Check sheet for the modelled part. Datum: model origin and axes. Units: mm. A direction names the side the tool comes from. Round coordinates to 2 decimals unless told otherwise and drop trailing zeros. Order: outer loops, then holes, each group sorted by start corner. A loop starts at its lowest first (then second) coordinate and runs counter-clockwise, first axis right, second up.
Q1. Cross-section at B-B on y = -12.5. Record the cut outline in (x, z), then the cut area to 3 significant figures.
Q2. Cross-section at A-A on x = 40. Record the cut outline in (y, z), then the cut area to 3 significant figures.
Q3. Scan lines: probe 1 along Z at (x, y) = (40, -13); probe 2 along Z at (x, y) = (42.5, -35.5); probe 3 along Z at (x, y) = (36.5, -9). Record each from-to range of solid material in increasing order.
Q4. Depth check by flat-ended pin: P1, Ø1.5, axis at x = 24, y = -31.5, coming from the -Z side; P2, Ø8, axis at x = 40, z = -24, coming from the -Y side; P3, Ø10, axis at x = 46.5, z = -14, coming from the -Y side; P4, Ø5, axis at x = 42.5, y = -30.5, coming from the -Z side. Enter the tip coordinate at first touch or a pass-through.
Q5. Mould release check, pull along X, two halves, no side actions. Record for faces 1 (the flat face through (26, -18, 0)), 2 (the cylindrical face through (0.86, -39.1, -15.72)), 3 (the cylindrical face through (36, -11, -27)): +X half, -X half, draft (parallel to the pull), parting line (faces both ways), or undercut.
Q6. Set-up check for faces 4 (the flat face through (54, -30, -11)), 5 (the cylindrical face through (54.1, -39.14, -6.01)): record each of +Z, -Z, +X, -X, +Y, -Y from which the full face is reachable in a straight line by a thin tool's end or side.
Q7. Cross-section at C-C on z = -24. Record the cut outline in (x, y), then the cut area to 3 significant figures.
Q8. Cross-section at D-D on y = -34.5. Record the cut outline in (x, z).
from build123d import *

# Parameters (mm, degrees)
F0_W         = 55
F0_H         = 32
F1_DEPTH     = 40
F2_W         = 30
F2_H         = 18
F3_DEPTH     = 20
F4_R         = 5
F5_DEPTH     = 22.001
F6_SIZE      = 2
F7_T1_DEPTH  = 36
F7_T3_DEPTH  = 45
F7_T5_DEPTH  = 68
F7_T7_DEPTH  = 23
F7_T12_DEPTH = 34.2132034356
F7_T17_DEPTH = 24.2132034356
F7_T22_DEPTH = 13.4214256026
F7_T29_DEPTH = 34.2132034356
F7_T33_DEPTH = 13.4214256026
F7_T40_DEPTH = 13.4214256026
F7_T44_DEPTH = 24.2132034356


# Not quite as in the source:
# - a fillet or chamfer that OpenCascade refuses, or shapes differently, is made with other operations: its cross-section is extruded or revolved along the edge and cut away or added


with BuildPart() as f1:
    # F0 (on Front) → F1 (new body)
    with BuildSketch(Plane.XZ):
        with Locations((27.5, -16)):
            Rectangle(F0_W, F0_H)
    extrude(amount=F1_DEPTH)

    # F2 (on face) → F3 (cut)
    with BuildSketch(Plane(origin=(0, 0, -32), x_dir=(1, 0, 0), z_dir=(0, 0, -1))):
        with Locations((40, 31)):
            Rectangle(F2_W, F2_H)
    extrude(amount=-F3_DEPTH, mode=Mode.SUBTRACT)

    # F4 (on face) → F5 (cut, through all)
    with BuildSketch(Plane.XZ.offset(22)):
        with Locations((40, -24)):
            Circle(F4_R)
    extrude(amount=-F5_DEPTH, mode=Mode.SUBTRACT)

    # F6
    f6_edges = [f1.edges().sort_by_distance(p)[0] for p in [
        (25, -40, -22),
        (25, -31, -32),
        (25, -31, -12),
        (55, -31, -12),
        (40, -40, -12),
        (55, -20, 0),
        (0, -20, -32),
    ]]
    chamfer(f6_edges, length=F6_SIZE)

    # F7: fillet of radius 3 on 7 edges, made by hand

    # F7_s2 → F7_t1 (cut)
    with BuildSketch(Plane.YZ.offset(-5.5)):
        with BuildLine():
            ThreePointArc((-40, -29), (-39.1213203436, -31.1213203436), (-37, -32))
            Line((-37, -32), (-40, -32))
            Line((-40, -32), (-40, -29))
        make_face()
    extrude(amount=F7_T1_DEPTH, mode=Mode.SUBTRACT)

    # F7_s4 → F7_t3 (cut)
    with BuildSketch(Plane.XY.offset(-37.5)):
        with BuildLine():
            ThreePointArc((0, -37), (0.8786796564, -39.1213203436), (3, -40))
            Line((3, -40), (0, -40))
            Line((0, -40), (0, -37))
        make_face()
    extrude(amount=F7_T3_DEPTH, mode=Mode.SUBTRACT)

    # F7_s6 → F7_t5 (cut)
    with BuildSketch(Plane.YZ.offset(-7.5)):
        with BuildLine():
            ThreePointArc((-37, 0), (-39.1213203436, -0.8786796564), (-40, -3))
            Line((-40, -3), (-40, 0))
            Line((-40, 0), (-37, 0))
        make_face()
    extrude(amount=F7_T5_DEPTH, mode=Mode.SUBTRACT)

    # F7_s8 → F7_t7 (cut)
    with BuildSketch(Plane.XY.offset(-17.5)):
        with BuildLine():
            ThreePointArc((52, -40), (54.1213203436, -39.1213203436), (55, -37))
            Line((55, -37), (55, -40))
            Line((55, -40), (52, -40))
        make_face()
    extrude(amount=F7_T7_DEPTH, mode=Mode.SUBTRACT)


with BuildPart() as f7_tool10:
    # F7_s11 → F7_t12 (new body)
    with BuildSketch(Plane.YZ.offset(58.1066017178)):
        with BuildLine():
            ThreePointArc((-40, -8.7573593129), (-39.7716385975, -9.90540961), (-39.1213203436, -10.8786796564))
            Line((-39.1213203436, -10.8786796564), (-40, -10))
            Line((-40, -10), (-40, -8.7573593129))
        make_face()
    extrude(amount=-F7_T12_DEPTH)

    split(bisect_by=Plane(origin=(25.6666666667, -25.6666666667, -25.6666666667), x_dir=(0.7071067812, 0.7071067812, 0), z_dir=(0.5773502692, -0.5773502692, -0.5773502692)), keep=Keep.TOP)


with BuildPart() as f1_1:
    add(f1.part)

    # F7_t9: cut F7_tool10
    add(f7_tool10.part, mode=Mode.SUBTRACT)


with BuildPart() as f7_tool15:
    # F7_s16 → F7_t17 (new body)
    with BuildSketch(Plane.XY.offset(-35.1066017178)):
        with BuildLine():
            ThreePointArc((21.7573593129, -40), (22.90540961, -39.7716385975), (23.8786796564, -39.1213203436))
            Line((23.8786796564, -39.1213203436), (23, -40))
            Line((23, -40), (21.7573593129, -40))
        make_face()
    extrude(amount=F7_T17_DEPTH)

    split(bisect_by=Plane(origin=(25.6666666667, -25.6666666667, -25.6666666667), x_dir=(0.7071067812, 0.7071067812, 0), z_dir=(0.5773502692, -0.5773502692, -0.5773502692)), keep=Keep.TOP)


with BuildPart() as f1_2:
    add(f1_1.part)

    # F7_t14: cut F7_tool15
    add(f7_tool15.part, mode=Mode.SUBTRACT)


with BuildPart() as f7_tool20:
    # F7_s21 → F7_t22 (new body)
    with BuildSketch(Plane(origin=(11.2451905284, 0, 11.2451905284), x_dir=(0, 1, 0), z_dir=(-0.7071067812, 0, -0.7071067812))):
        with BuildLine():
            ThreePointArc((-40, 24.6100366333), (-39.6642215019, 25.9891391634), (-38.7320508076, 27.0595263761))
            Line((-38.7320508076, 27.0595263761), (-40, 26.1629509039))
            Line((-40, 26.1629509039), (-40, 24.6100366333))
        make_face()
    extrude(amount=F7_T22_DEPTH)

    split(bisect_by=Plane(origin=(0, -25, -25), x_dir=(1, 0, 0), z_dir=(0, -0.7071067812, -0.7071067812)), keep=Keep.TOP)

    split(bisect_by=Plane(origin=(31.5, -31.5, 0), x_dir=(0, 0, 1), z_dir=(0.7071067812, -0.7071067812, 0)), keep=Keep.TOP)


with BuildPart() as f1_3:
    add(f1_2.part)

    # F7_t19: cut F7_tool20
    add(f7_tool20.part, mode=Mode.SUBTRACT)


with BuildPart() as f7_tool27:
    # F7_s28 → F7_t29 (new body)
    with BuildSketch(Plane.YZ.offset(58.1066017178)):
        with BuildLine():
            ThreePointArc((-40, -8.7573593129), (-39.7716385975, -9.90540961), (-39.1213203436, -10.8786796564))
            Line((-39.1213203436, -10.8786796564), (-40, -10))
            Line((-40, -10), (-40, -8.7573593129))
        make_face()
    extrude(amount=-F7_T29_DEPTH)

    split(bisect_by=Plane(origin=(25.6666666667, -25.6666666667, -25.6666666667), x_dir=(-0.7071067812, -0.7071067812, 0), z_dir=(-0.5773502692, 0.5773502692, 0.5773502692)), keep=Keep.TOP)


with BuildPart() as f7_tool31:
    # F7_s32 → F7_t33 (new body)
    with BuildSketch(Plane(origin=(11.2451905284, 0, 11.2451905284), x_dir=(0, 1, 0), z_dir=(-0.7071067812, 0, -0.7071067812))):
        with BuildLine():
            ThreePointArc((-40, 24.6100366333), (-39.6642215019, 25.9891391634), (-38.7320508076, 27.0595263761))
            Line((-38.7320508076, 27.0595263761), (-40, 26.1629509039))
            Line((-40, 26.1629509039), (-40, 24.6100366333))
        make_face()
    extrude(amount=F7_T33_DEPTH)

    split(bisect_by=Plane(origin=(0, -25, -25), x_dir=(1, 0, 0), z_dir=(0, 0.7071067812, 0.7071067812)), keep=Keep.TOP)


with BuildPart() as f7_tool27_1:
    add(f7_tool27.part)

    # F7_t35: intersect F7_tool31
    add(f7_tool31.part, mode=Mode.INTERSECT)


with BuildPart() as f1_4:
    add(f1_3.part)

    # F7_t25: cut F7_tool27
    add(f7_tool27_1.part, mode=Mode.SUBTRACT)


with BuildPart() as f7_tool38:
    # F7_s39 → F7_t40 (new body)
    with BuildSketch(Plane(origin=(11.2451905284, 0, 11.2451905284), x_dir=(0, 1, 0), z_dir=(-0.7071067812, 0, -0.7071067812))):
        with BuildLine():
            ThreePointArc((-40, 24.6100366333), (-39.6642215019, 25.9891391634), (-38.7320508076, 27.0595263761))
            Line((-38.7320508076, 27.0595263761), (-40, 26.1629509039))
            Line((-40, 26.1629509039), (-40, 24.6100366333))
        make_face()
    extrude(amount=F7_T40_DEPTH)

    split(bisect_by=Plane(origin=(31.5, -31.5, 0), x_dir=(0, 0, 1), z_dir=(-0.7071067812, 0.7071067812, 0)), keep=Keep.TOP)


with BuildPart() as f7_tool42:
    # F7_s43 → F7_t44 (new body)
    with BuildSketch(Plane.XY.offset(-35.1066017178)):
        with BuildLine():
            ThreePointArc((21.7573593129, -40), (22.90540961, -39.7716385975), (23.8786796564, -39.1213203436))
            Line((23.8786796564, -39.1213203436), (23, -40))
            Line((23, -40), (21.7573593129, -40))
        make_face()
    extrude(amount=F7_T44_DEPTH)

    split(bisect_by=Plane(origin=(25.6666666667, -25.6666666667, -25.6666666667), x_dir=(-0.7071067812, -0.7071067812, 0), z_dir=(-0.5773502692, 0.5773502692, 0.5773502692)), keep=Keep.TOP)


with BuildPart() as f7_tool38_1:
    add(f7_tool38.part)

    # F7_t46: intersect F7_tool42
    add(f7_tool42.part, mode=Mode.INTERSECT)


with BuildPart() as f1_5:
    add(f1_4.part)

    # F7_t36: cut F7_tool38
    add(f7_tool38_1.part, mode=Mode.SUBTRACT)


solid = f1_5.part
Results found:
1. outline: (0, -30) - (2, -32) - (55, -32) - (55, -2) - (53, 0) - (0, 0) - close; hole circle Ø10 at (40, -24)
1. area: 1,680 mm2
2. outline: (-40, -8.76) arc R3 ccw to (-39.12, -10.88) - (-38, -12) - (-22, -12) - (-22, -19) - (0, -19) - (0, 0) - (-37, 0) arc R3 ccw to (-40, -3) - close; (-22, -32) - (0, -32) - (0, -29) - (-22, -29) - close
2. area: 696 mm2
3. probe 1: z = -32 to -29, -19 to 0
3. probe 2: z = -12 to 0
3. probe 3: z = -32 to -27.57, -20.43 to 0
4. P1: stops at z = -31.75
4. P2: passes through
4. P3: stops at y = -39.99
4. P4: stops at z = -12
5. face 1: draft
5. face 2: -X half
5. face 3: undercut
6. face 4: -Z, +X, -Y
6. face 5: +Z, -Z, +X, -Y
7. outline: (0, -37) arc R3 ccw to (3, -40) - (21.76, -40) arc R3 ccw to (23.88, -39.12) - (25, -38) - (25, -22) - (35, -22) - (35, 0) - (0, 0) - close; (45, -22) - (55, -22) - (55, 0) - (45, 0) - close
7. area: 1,440 mm2
8. outline: (0, -30) - (2, -32) - (23, -32) - (25, -30) - (25, -14) - (27, -12) - (53, -12) - (55, -10) - (55, -2) - (53, 0) - (0, 0) - close
